Could you check a few things on this model? Use its own coordinates, in mm. A direction names the side the tool comes from. Give positions to 0.01 mm unless a question says otherwise; leave off trailing zeros. Write each loop counter-clockwise with the first axis right and the second up, starting at its lowest first coordinate (ties: lowest second). Pieces come first, ordered by that corner, then holes. Notation, with made-up numbers: M 40.25,-29 L 67.25,-29 A25 cw 67.25,-12 Z; hole C 3.5,33 d10. An arc over 180 degrees is marked long. Answer as CSV lines item,"result". Start each with the question number.
from build123d import *

# Parameters (mm, degrees)
SKETCH_1_R           = 2.85
EXTRUDE_1_DEPTH      = 31
SKETCH_3_W           = 5.9
SKETCH_3_H           = 5.9
EXTRUDE_2_DEPTH      = 5
SKETCH_4_R           = 5
EXTRUDE_3_DEPTH      = 7
SKETCH_6_R           = 11.5
EXTRUDE_4_DEPTH      = 2
SKETCH_8_R           = 4.5
CUT_EXTRUDE_2_DEPTH  = 7.5
SKETCH_9_R           = 1.25
CUT_EXTRUDE_3_DEPTH  = 5.5
SKETCH_10_R          = 1.175
CUT_EXTRUDE_7_DEPTH  = 10
SKETCH_12_W          = 5.9
SKETCH_12_H          = 5.9
EXTRUDE_5_DEPTH      = 45
SKETCH_15_W          = 5.9
SKETCH_15_H          = 20.04910328
EXTRUDE_6_DEPTH      = 6
SKETCH_16_R          = 1.175
CUT_EXTRUDE_8_DEPTH  = 10
SKETCH_21_W          = 41.5
SKETCH_21_H          = 3.1
CUT_EXTRUDE_9_DEPTH  = 10
SKETCH_22_OUTSIDE_W  = 45.272
SKETCH_22_OUTSIDE_H  = 45.272
SKETCH_22_OUTSIDE_R  = 2.85
CUT_EXTRUDE_10_DEPTH = 5
SKETCH_23_R          = 14.411618967
CUT_EXTRUDE_11_DEPTH = 9


with BuildPart() as part:
    # 스케치1 → 보스-돌출1 (new body)
    with BuildSketch(Plane.XY):
        Circle(SKETCH_1_R)
    extrude(amount=EXTRUDE_1_DEPTH)

    # 스케치3 → 보스-돌출2 (add)
    with BuildSketch(Plane(origin=(0, 0, 0), x_dir=(-1, 0, 0), z_dir=(0, 0, -1))):
        Rectangle(SKETCH_3_W, SKETCH_3_H)
    extrude(amount=EXTRUDE_2_DEPTH)

    # 스케치4 → 보스-돌출3 (add)
    with BuildSketch(Plane(origin=(0, 0, -5), x_dir=(-1, 0, 0), z_dir=(0, 0, -1))):
        Circle(SKETCH_4_R)
    extrude(amount=EXTRUDE_3_DEPTH)

    # 스케치6 → 보스-돌출4 (add)
    with BuildSketch(Plane(origin=(0, 0, -12), x_dir=(-1, 0, 0), z_dir=(0, 0, -1))):
        Circle(SKETCH_6_R)
    extrude(amount=EXTRUDE_4_DEPTH)

    # 스케치8 → 컷-돌출2 (cut)
    with BuildSketch(Plane(origin=(0, 0, -14), x_dir=(-1, 0, 0), z_dir=(0, 0, -1))):
        Circle(SKETCH_8_R)
    extrude(amount=-CUT_EXTRUDE_2_DEPTH, mode=Mode.SUBTRACT)

    # 스케치9 → 컷-돌출3 (cut)
    with BuildSketch(Plane(origin=(0, 0, -14), x_dir=(-1, 0, 0), z_dir=(0, 0, -1))):
        with Locations((3.444150891, 8.314915793)):
            Circle(SKETCH_9_R)
        with Locations((-3.444150891, 8.314915793)):
            Circle(SKETCH_9_R)
        with Locations((8.314915793, 3.444150891)):
            Circle(SKETCH_9_R)
        with Locations((8.314915793, -3.444150891)):
            Circle(SKETCH_9_R)
        with Locations((3.444150891, -8.314915793)):
            Circle(SKETCH_9_R)
        with Locations((-3.444150891, -8.314915793)):
            Circle(SKETCH_9_R)
        with Locations((-8.314915793, -3.444150891)):
            Circle(SKETCH_9_R)
        with Locations((-8.314915793, 3.444150891)):
            Circle(SKETCH_9_R)
    extrude(amount=-CUT_EXTRUDE_3_DEPTH, mode=Mode.SUBTRACT)

    # 스케치10 → 컷-돌출7 (cut)
    with BuildSketch(Plane(origin=(0, 2.95, 0), x_dir=(1, 0, 0), z_dir=(0, 1, 0))):
        with Locations(Location((0, 2.2, 0), (0, 0, 180))):
            Circle(SKETCH_10_R)
    extrude(amount=-CUT_EXTRUDE_7_DEPTH, mode=Mode.SUBTRACT)

    # 스케치12 → 보스-돌출5 (add)
    with BuildSketch(Plane.XY.offset(31)):
        Rectangle(SKETCH_12_W, SKETCH_12_H)
    extrude(amount=EXTRUDE_5_DEPTH)

    # 스케치15 → 보스-돌출6 (add)
    with BuildSketch(Plane.XY.offset(76)):
        Rectangle(SKETCH_15_W, SKETCH_15_H)
    extrude(amount=EXTRUDE_6_DEPTH)

    # 스케치16 → 컷-돌출8 (cut)
    with BuildSketch(Plane(origin=(0, 2.95, 0), x_dir=(1, 0, 0), z_dir=(0, 1, 0))):
        with Locations(Location((0, -33.2, 0), (0, 0, 270))):
            Circle(SKETCH_16_R)
    extrude(amount=-CUT_EXTRUDE_8_DEPTH, mode=Mode.SUBTRACT)

    # 스케치21 → 컷-돌출9 (cut)
    with BuildSketch(Plane(origin=(2.95, 0, 0), x_dir=(0, 0, -1), z_dir=(1, 0, 0))):
        with Locations((-15.75, 1.4)):
            Rectangle(SKETCH_21_W, SKETCH_21_H)
    extrude(amount=-CUT_EXTRUDE_9_DEPTH, mode=Mode.SUBTRACT)

    # 스케치22 outside → 컷-돌출10 (cut)
    with BuildSketch(Plane.XY):
        Rectangle(SKETCH_22_OUTSIDE_W, SKETCH_22_OUTSIDE_H)
        Circle(SKETCH_22_OUTSIDE_R, mode=Mode.SUBTRACT)
    extrude(amount=-CUT_EXTRUDE_10_DEPTH, mode=Mode.SUBTRACT)

    # 스케치23 → 컷-돌출11 (cut)
    with BuildSketch(Plane(origin=(0, 0, -14), x_dir=(-1, 0, 0), z_dir=(0, 0, -1))):
        Circle(SKETCH_23_R)
    extrude(amount=-CUT_EXTRUDE_11_DEPTH, mode=Mode.SUBTRACT)


solid = part.part
1. Imagine slicing it at D-D, the plane y = 7.75. Please give me the cut outline in (x, z), plus the area to 3 significant figures.
2. Imagine slicing it at C-C, the plane y = 1.25. Please give me the cut outline in (x, z).
3. On a 3-axis mill with a long thin cutter (end or side, diameter ignored), from which of +Z, -Z, +X, -X, +Y, -Y can I reach the whole of each face in a straight line? I mean faces 1 (the flat face through (2.95, 0, 62)), 2 (the flat face through (0, 2.95, 56)), 3 (the cylindrical face through (-0.06, -2.85, 12.75)), 4 (the cylindrical face through (0.052, -1.53, 32.026)), 5 (the flat face through (0, -2.95, 53)). Say none if no direction works.
4. Imagine slicing it at B-B, the plane z = 33.2. Please give me the cut outline in (x, y) (3 decimals).
5. Imagine slicing it at A-A, the plane x = 0. Please give me the cut outline in (y, z) (3 decimals).
6. Thinking about a two-plate mould opening in X: for faces 6 (the cylindrical face through (1.174, -1.483, -2.148)), 7 (the flat face through (-2.95, 0, 62)), 8 (the flat face through (0, -0.15, 16)), which applies, pulls with the +X half, pulls with the -X half, needs draft (parallel to the pull), parting line crosses it, or undercut?
7. Please list where these lines run through material, in increasing order: line 1 (X direction, y = -2.3, z = 33.2) (3 decimals); line 2 (Z direction, x = 2.5, y = -6.5); line 3 (Y direction, x = -0.5, z = 56.5).
8. Will these pins go through, and if not, where does the flat tip stop? P1, Ø1.5, axis at x = -1.5, z = 40.5, coming from the +Y side; P2, Ø2, axis at x = 0, z = 33.2, coming from the -Y side.
Solutions:
1,outline,"M -2.95,76 L 2.95,76 L 2.95,82 L -2.95,82 Z"
1,area,"35.4 mm²"
2,outline,"M -2.95,36.5 L 2.95,36.5 L 2.95,82 L -2.95,82 Z"
3,face 1,"+Z, -Z, +X, +Y, -Y"
3,face 2,"-Z, +X, -X, +Y"
3,face 3,"-Z, -Y"
3,face 4,"+Y, -Y"
3,face 5,"-Z, +X, -X, -Y"
4,outline,"M -2.95,-2.95 L -1.175,-2.95 L -1.175,-0.15 L -2.95,-0.15 Z; M 1.175,-2.95 L 2.95,-2.95 L 2.95,-0.15 L 1.175,-0.15 Z"
5,outline,"M -10.025,76 L -2.95,76 L -2.95,34.375 L -0.15,34.375 L -0.15,36.5 L 2.95,36.5 L 2.95,76 L 10.025,76 L 10.025,82 L -10.025,82 Z; M -2.95,31 L -2.85,31 L -2.85,-1.025 L -0.15,-1.025 L -0.15,32.025 L -2.95,32.025 Z; M -2.85,-5 L -0.15,-5 L -0.15,-3.375 L -2.85,-3.375 Z"
6,face 6,"undercut"
6,face 7,"pulls with the -X half"
6,face 8,"needs draft"
7,line 1,"-2.95 to -1.175, 1.175 to 2.95"
7,line 2,"76 to 82"
7,line 3,"-2.95 to 2.95"
8,P1,"y = 2.95"
8,P2,"through"
